Part print with two shaded views. Sizes in mm from the minimum x, y, z corner. A direction names the side the tool comes from. Round coordinates to 2 decimals unless told otherwise and drop trailing zeros. Order: outer loops, then holes, each group sorted by start corner. A loop starts at its lowest first (then second) coordinate and runs counter-clockwise, first axis right, second up. Notation, with made-up numbers: M 69.25,9 L 94.25,9 A27 ccw 94.25,30 Z; hole C 26.25,-21 d3. An arc over 180 degrees is marked long. Answer as a JSON object with one key per item and string values.
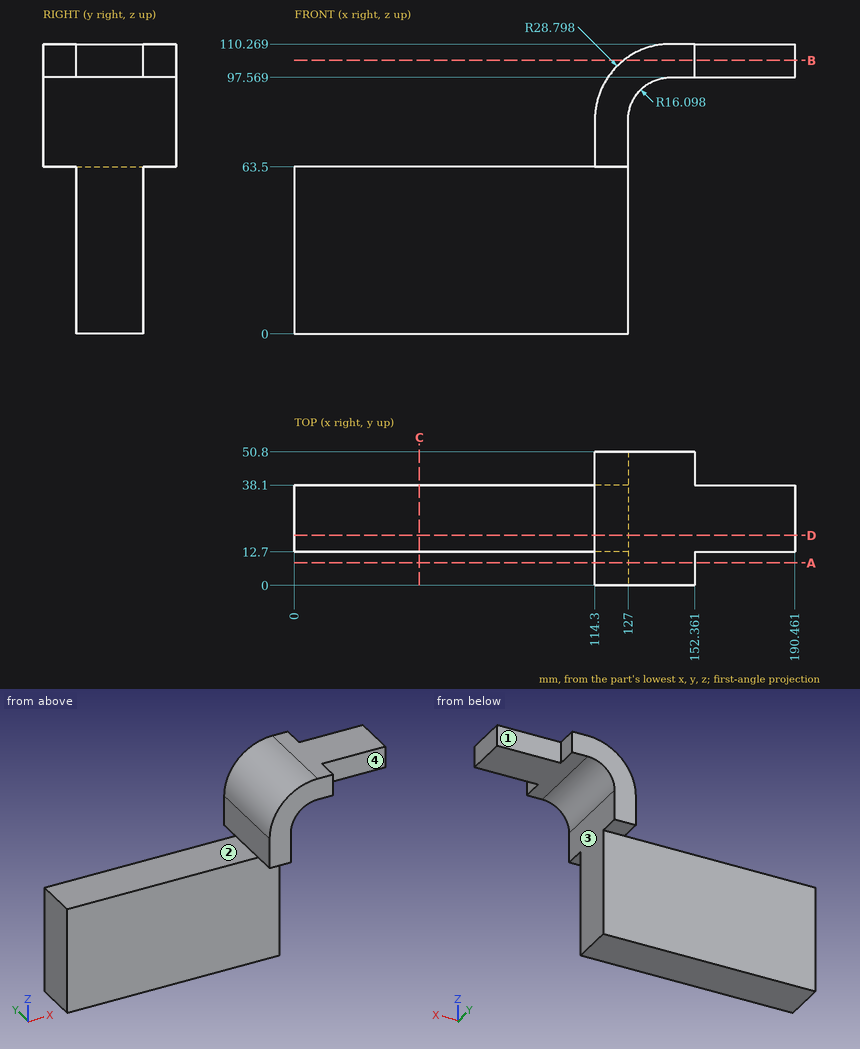
Item 1: Saw through at A-A on y = 8.5. List the corners of the cut face in (x, z) (1 decimal), and give its area (3 significant figures).
Worked answers:
{"outline": "M 114.3,63.5 L 127,63.5 L 127,81.5 A16.1 cw 143.1,97.6 L 152.4,97.6 L 152.4,110.3 L 143.1,110.3 A28.8 ccw 114.3,81.5 Z", "area": "794 mm2"}
Item 2: Saw through at C-C on x = 47.5. List the corners of the cut face in (y, z), and give its area (3 significant figures).
Worked answers:
{"outline": "M 12.7,0 L 38.1,0 L 38.1,63.5 L 12.7,63.5 Z", "area": "1,610 mm2"}
Item 3: Drop flat-ended pins along their axis: pin 1 Ø12.5 at (x, y) = (72.5, 31) entering from +Z; pin 2 Ø14 at (x, y) = (178, 16.5) entering from -Z; pin 3 Ø10 at (x, z) = (172.5, 105.5) entering from -Y. Give the stop position or say it passes through.
Worked answers:
{"pin 1": "stops at z = 63.5", "pin 2": "stops at z = 97.57", "pin 3": "stops at y = 12.7"}
Item 4: Saw through at D-D on y = 19. List the corners of the cut face in (x, z) (1 decimal), and give its area (3 significant figures).
Worked answers:
{"outline": "M 0,0 L 127,0 L 127,81.5 A16.1 cw 143.1,97.6 L 190.5,97.6 L 190.5,110.3 L 143.1,110.3 A28.8 ccw 114.3,81.5 L 114.3,63.5 L 0,63.5 Z", "area": "9,340 mm2"}
Item 5: 3-axis set-ups, long thin cutter, end or side, ignore diameter. For the marked faces 1, 2, 3 and 4: which of +Z, -Z, +X, -X, +Y, -Y reach the whole face in a straight line?
Worked answers:
{"face 1": "+Z, -Z, +X, +Y", "face 2": "+Z, -X, +Y, -Y", "face 3": "-Z, +X, +Y, -Y", "face 4": "+Z, -Z, +X, -Y"}
Item 6: Wall check: line 1 along X through (y, z) = (22, 39); line 2 along X through (y, z) = (40, 66.5); line 3 along Z through (x, y) = (152, 17). Give the ranges that are in metal, low to high. Write a range as [from, to].
Worked answers:
{"line 1": "x = [0, 127]", "line 2": "x = [114.3, 127]", "line 3": "z = [97.57, 110.27]"}
Item 7: Saw through at B-B on z = 104. List the corners of the cut face in (x, y), and give its area (3 significant figures).
Worked answers:
{"outline": "M 125.16,0 L 152.36,0 L 152.36,12.7 L 190.46,12.7 L 190.46,38.1 L 152.36,38.1 L 152.36,50.8 L 125.16,50.8 Z", "area": "2,350 mm2"}
